Could you check a few things on this drawing? It's one solid part, dimensions in mm from its lowest x, y, z. Coordinates: 2 decimals unless noted, no trailing zeros. Return JSON: item names as keys, results as strings. Group by question number.
1) If I drill on line 1 along X through (y, z) = (89, 17.5) (1 decimal); line 2 along Y through (x, z) = (271.5, 5) (1 decimal); line 3 along X through (y, z) = (63.5, 4), over which ranges is the centre line in solid material (lowest first)?
2) Imagine slicing it at A-A (y = 84). Give the number of separate pieces and of enclosed holes in the cut face, and give its area (3 significant figures).
3) For pin 1 Ø4 at (y, z) = (212, 8.5) entering from -X, with a flat end and sliding along its axis, tell me the tip position at first contact or that it passes through.
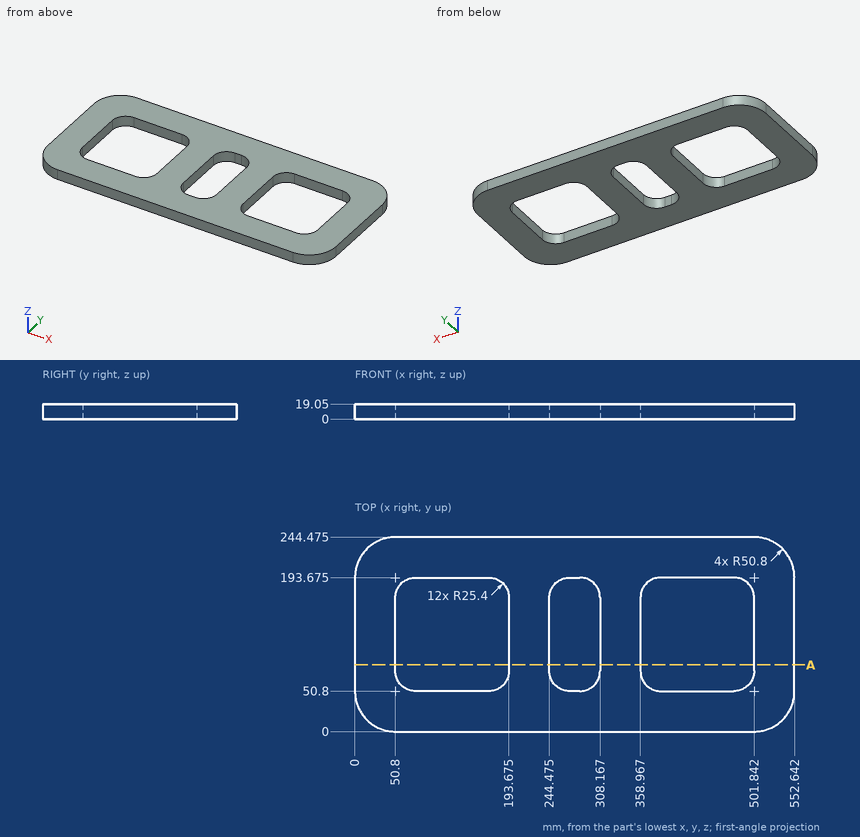
Calculated:
{
 "1": {"line 1": "0 to 50.8, 193.7 to 244.5, 308.2 to 359, 501.8 to 552.6", "line 2": "0 to 50.8, 193.7 to 244.5", "line 3": "0 to 54.2, 190.27 to 247.88, 304.76 to 362.37, 498.44 to 552.64"},
 "2": {"separate pieces": "4", "enclosed holes": "0", "area": "3,870 mm2"},
 "3": {"pin 1": "x = 2.69"}
}
